Solid Edge part; units mm, degrees
sketch "Sketch1" plane through (0, 0, 0) normal (0, 0, 1) x (1, 0, 0)
  line L0 (-40, -40) -> (40, -40)
  line L1 (40, -40) -> (40, 40)
  line L2 (40, 40) -> (-40, 40)
  line L3 (-40, 40) -> (-40, -40)
extrude "Extrusionsausprägung_20" add sketch "Sketch1" along normal blind 8
sketch "Sketch2" plane through (0, 0, 0) normal (0, 0, 1) x (1, 0, 0)
  circle A0 centre (0, 0) radius 13
extrude "Extrusionsausschnitt_24" cut sketch "Sketch2" along normal blind 6
sketch "Sketch3" plane through (0, 0, 6) normal (0, 0, -1) x (1, 0, 0)
  circle A0 centre (0, 0) radius 10
extrude "Extrusionsausschnitt_25" cut sketch "Sketch3" against normal blind 140
sketch "Sketch4" plane through (0, 0, 0) normal (0, 0, -1) x (1, 0, 0)
  circle A0 centre (-30, 30) radius 6.5
  circle A1 centre (30, 30) radius 6.5
  circle A2 centre (30, -30) radius 6.5
  circle A3 centre (-30, -30) radius 6.5
extrude "Extrusionsausschnitt_26" cut sketch "Sketch4" against normal blind 59
sketch "Sketch5" plane through (0, 0, 0) normal (0, 0, -1) x (1, 0, 0)
  line L0 (10, 70) -> (-10, 70)
  line L1 (-10, 70) -> (-10, 40)
  line L2 (-10, 40) -> (10, 40)
  line L3 (10, 40) -> (10, 70)
extrude "Protrusion1" add sketch "Sketch5" against normal up to vertex (8 mm away)
fillet "Verrundung_15" radius 10 2 edges at (10, -70, 4) (-10, -70, 4)
fillet "Verrundung_16" radius 1 2 edges at (10, -40, 4) (-10, -40, 4)
mirror "Mirror1" about plane through (0, 0, 0) normal (0, -1, 0) of "Protrusion1", "Verrundung_15", "Verrundung_16"
hole "Bohrung_4" at (-17.5, -17.5, 0) direction (0, 0, 1) diameter 3.3 end up to next
hole "Hole1" at (17.5, -17.5, 0) direction (0, 0, 1) diameter 3.3 end up to next
hole "Hole2" at (17.5, 17.5, 0) direction (0, 0, 1) diameter 3.3 end up to next
hole "Hole3" at (-17.5, 17.5, 0) direction (0, 0, 1) diameter 3.3 end up to next
fillet "Verrundung_17" radius 5 4 edges at (-40, -40, 4) (40, -40, 4) (-40, 40, 4) (40, 40, 4)
chamfer "Fase_9" distance 1 angle 45 29 edges at (-17.5, 19.15, 0) (17.5, 19.15, 0) (17.5, -15.85, 0) (-17.5, -15.85, 0) (-36.5, -30, 0) (23.5, -30, 0) (23.5, 30, 0) (-36.5, 30, 0) (-13, 0, 0) (23, 40, 0) (38.5355, 38.5355, 0) (40, 0, 0) (38.5355, -38.5355, 0) (23, -40, 0) (10.2929, -40.2929, 0) (10, -50.5, 0) (0, -70, 0) (-10, -50.5, 0) (-10.2929, -40.2929, 0) (-23, -40, 0) (-38.5355, -38.5355, 0) (-40, 0, 0) (-38.5355, 38.5355, 0) (-23, 40, 0) (-10.2929, 40.2929, 0) (-10, 50.5, 0) (0, 70, 0) (10, 50.5, 0) (10.2929, 40.2929, 0)
chamfer "Fase_10" distance 1 angle 45 29 edges at (-19.15, 17.5, 8) (15.85, 17.5, 8) (15.85, -17.5, 8) (-19.15, -17.5, 8) (-36.5, -30, 8) (23.5, -30, 8) (23.5, 30, 8) (-36.5, 30, 8) (-10, 0, 8) (40, 0, 8) (38.5355, 38.5355, 8) (23, 40, 8) (10.2929, 40.2929, 8) (10, 50.5, 8) (0, 70, 8) (-10, 50.5, 8) (-10.2929, 40.2929, 8) (-23, 40, 8) (-38.5355, 38.5355, 8) (-40, 0, 8) (-38.5355, -38.5355, 8) (-23, -40, 8) (-10.2929, -40.2929, 8) (-10, -50.5, 8) (0, -70, 8) (10, -50.5, 8) (10.2929, -40.2929, 8) (23, -40, 8) (38.5355, -38.5355, 8)
For this review, take the finished solid that the model builds, in its own axes (mm). A direction names the side the tool comes from. Coordinates: 2 decimals unless noted, no trailing zeros. Order: outer loops, then holes, each group sorted by start corner. A loop starts at its lowest first (then second) coordinate and runs counter-clockwise, first axis right, second up. Notation, with made-up numbers: (29, -16) - (45, -16) arc R18 cw to (45, -10) - close; hole circle Ø4 at (66.25, 88). An arc over 180 degrees is marked (long way). Answer as a JSON object with one key per item and string values. Group by question number.
1. For faces 4 (the cylindrical face through (29.154, -36.445, 3.958)), 5 (the flat face through (23, 40, 4)), 6 (the flat face through (23, -40, 4)), list the 3-axis set-ups (+Z, -Z, +X, -X, +Y, -Y) from which the entire face can be reached by the end or side of a thin tool; tool diameter is ignored.
2. We need section C-C on z = 4.5. Give the number of separate pieces and of enclosed holes in the cut face, then the cut area to 3 significant figures.
3. The part is to be moulded in two halves that separate along X. For faces 1 (the conical face through (-37.996, -38.063, 7.715)), 2 (the flat face through (7, -8, 6)), 3 (the flat face through (-23, -40, 4)), say which applies: pulls with the +X half, pulls with the -X half, needs draft (parallel to the pull), parting line crosses it, or undercut.
4. For probe 1 along Y at (x, z) = (30, 3.2); probe 2 along Y at (x, z) = (-17.5, 2.9), list the stretches that pass through material, from the lowest coordinate up.
5. We need section D-D on y = 52. State the section outline as (x, z) points, then the cut area to 3 significant figures.
6. We need section A-A on x = -30. State the section outline as (y, z) points, then the cut area to 3 significant figures.
7. Clearance check with flat-ended pins moving along their axes: P1, Ø3, axis at y = 47, z = 4, coming from the +X side; P2, Ø1.8, axis at y = 46.5, z = 3.5, coming from the -X side; P3, Ø4.5, axis at x = 17.5, y = -17.5, coming from the -Z side; P4, Ø21, axis at x = -30, y = -30, coming from the +Z side. State where each tip first meets the part, or that it passes through.
Final values:
{
 "1": {"face 4": "+Z, -Z", "face 5": "+Z, -Z, +X, +Y", "face 6": "+Z, -Z, +X, -Y"},
 "2": {"separate pieces": "1", "enclosed holes": "9", "area": "6,400 mm²"},
 "3": {"face 1": "pulls with the -X half", "face 2": "undercut", "face 3": "needs draft"},
 "4": {"probe 1": "-40 to -36.5, -23.5 to 23.5, 36.5 to 40", "probe 2": "-40 to -19.15, -15.85 to 15.85, 19.15 to 40"},
 "5": {"outline": "(-10, 1) - (-9, 0) - (9, 0) - (10, 1) - (10, 7) - (9, 8) - (-9, 8) - (-10, 7) - close", "area": "158 mm²"},
 "6": {"outline": "(-40, 1) - (-39, 0) - (-37.5, 0) - (-36.5, 1) - (-36.5, 7) - (-37.5, 8) - (-39, 8) - (-40, 7) - close; (-23.5, 1) - (-22.5, 0) - (22.5, 0) - (23.5, 1) - (23.5, 7) - (22.5, 8) - (-22.5, 8) - (-23.5, 7) - close; (36.5, 1) - (37.5, 0) - (39, 0) - (40, 1) - (40, 7) - (39, 8) - (37.5, 8) - (36.5, 7) - close", "area": "426 mm²"},
 "7": {"P1": "x = 10", "P2": "x = -10", "P3": "z = 0.4", "P4": "z = 8"}
}
